from build123d import *
from OCP.BRepFilletAPI import BRepFilletAPI_MakeChamfer

# Parameters (mm, degrees)
SKETCH_1_W      = 20.2
SKETCH_1_H      = 50
SKETCH_1_R      = 1.325
SKETCH_1_R_2    = 1.595
SKETCH_1_W_2    = 6
SKETCH_1_H_2    = 10.9
EXTRUDE_1_DEPTH = 2
FILLET_1_R      = 2
CHAMFER_1_SIZE  = 0.6
CHAMFER_2_SIZE  = 0.5
CHAMFER_2_SIZE2 = 0.595876796


with BuildPart() as part:
    # 草图1 → 凸台-拉伸1 (new body)
    with BuildSketch(Plane.XY):
        with Locations((-6.4, 0)):
            Rectangle(SKETCH_1_W, SKETCH_1_H)
        with Locations((-14.25, -22.65)):
            Circle(SKETCH_1_R, mode=Mode.SUBTRACT)
        with Locations((-14.25, 22.65)):
            Circle(SKETCH_1_R, mode=Mode.SUBTRACT)
        with Locations((1.45, 22.65)):
            Circle(SKETCH_1_R, mode=Mode.SUBTRACT)
        with Locations((1.45, -22.65)):
            Circle(SKETCH_1_R, mode=Mode.SUBTRACT)
        with Locations((-10.36, -6.365)):
            Circle(SKETCH_1_R_2, mode=Mode.SUBTRACT)
        with Locations((-10.36, -11.8216)):
            Circle(SKETCH_1_R_2, mode=Mode.SUBTRACT)
        with Locations((-4.095, 6)):
            Rectangle(SKETCH_1_W_2, SKETCH_1_H_2, mode=Mode.SUBTRACT)
    extrude(amount=EXTRUDE_1_DEPTH)

    # 圆角1
    fillet_1_edges = [part.edges().sort_by_distance(p)[0] for p in [
        (-16.5, 25, 1),
        (3.7, 25, 1),
        (3.7, -25, 1),
        (-16.5, -25, 1),
    ]]
    fillet(fillet_1_edges, radius=FILLET_1_R)

    # 倒角1
    chamfer_1_edges = [part.edges().sort_by_distance(p)[0] for p in [
        (-15.575, -22.65, 2),
        (-15.575, 22.65, 2),
        (0.125, 22.65, 2),
        (0.125, -22.65, 2),
    ]]
    chamfer(chamfer_1_edges, length=CHAMFER_1_SIZE)

    # 倒角2: one chamfer whose edges measure the first distance from different faces: ONE call of the kernel's chamfer builder (chamfer() names one face for all edges)
    chamfer_2_edges_1 = [part.edges().sort_by_distance(p)[0] for p in [
        (-7.095, 6, 0),
        (-7.095, 11.45, 1),
        (-7.095, 0.55, 1),
        (-7.095, 6, 2),
    ]]
    chamfer_2_side_1 = [part.faces().sort_by_distance(p)[0] for p in [
        (-7.095, 6, 1),
    ]]
    chamfer_2_edges_2 = [part.edges().sort_by_distance(p)[0] for p in [
        (-4.095, 0.55, 0),
    ]]
    chamfer_2_side_2 = [part.faces().sort_by_distance(p)[0] for p in [
        (-4.095, 0.55, 1),
    ]]
    chamfer_2_edges_3 = [part.edges().sort_by_distance(p)[0] for p in [
        (-1.095, 6, 0),
        (-1.095, 0.55, 1),
    ]]
    chamfer_2_side_3 = [part.faces().sort_by_distance(p)[0] for p in [
        (-1.095, 6, 1),
    ]]
    chamfer_2_edges_4 = [part.edges().sort_by_distance(p)[0] for p in [
        (-4.095, 11.45, 0),
        (-1.095, 11.45, 1),
    ]]
    chamfer_2_side_4 = [part.faces().sort_by_distance(p)[0] for p in [
        (-4.095, 11.45, 1),
    ]]
    chamfer_2_edges_5 = [part.edges().sort_by_distance(p)[0] for p in [
        (-4.095, 0.55, 2),
        (-1.095, 6, 2),
        (-4.095, 11.45, 2),
    ]]
    chamfer_2_side_5 = [part.faces().sort_by_distance(p)[0] for p in [
        (-6.499529382, -0.281178063, 2),
    ]]
    chamfer_2 = BRepFilletAPI_MakeChamfer(part.part.solid().wrapped)
    for e in chamfer_2_edges_1:
        chamfer_2.Add(CHAMFER_2_SIZE, CHAMFER_2_SIZE2, e.wrapped, chamfer_2_side_1[0].wrapped)  # the first distance lies on this face
    for e in chamfer_2_edges_2:
        chamfer_2.Add(CHAMFER_2_SIZE, CHAMFER_2_SIZE2, e.wrapped, chamfer_2_side_2[0].wrapped)  # the first distance lies on this face
    for e in chamfer_2_edges_3:
        chamfer_2.Add(CHAMFER_2_SIZE, CHAMFER_2_SIZE2, e.wrapped, chamfer_2_side_3[0].wrapped)  # the first distance lies on this face
    for e in chamfer_2_edges_4:
        chamfer_2.Add(CHAMFER_2_SIZE, CHAMFER_2_SIZE2, e.wrapped, chamfer_2_side_4[0].wrapped)  # the first distance lies on this face
    for e in chamfer_2_edges_5:
        chamfer_2.Add(CHAMFER_2_SIZE, CHAMFER_2_SIZE2, e.wrapped, chamfer_2_side_5[0].wrapped)  # the first distance lies on this face
    add(Compound.cast(chamfer_2.Shape()), mode=Mode.REPLACE)


solid = part.part
Here's how the part is built. I have some questions about the finished solid (model axes, mm). A direction names the side the tool comes from. Round coordinates to 2 decimals unless told otherwise and drop trailing zeros. Order: outer loops, then holes, each group sorted by start corner. A loop starts at its lowest first (then second) coordinate and runs counter-clockwise, first axis right, second up. Notation, with made-up numbers: (89.25, -40) -> (126.25, -40) arc R11 cw to (126.25, -26) -> close; hole circle Ø6 at (33.25, 49.25). An arc over 180 degrees is marked (long way). Use CSV: the item, a comma, the result in double quotes.
1. I'm going to push a flat-ended pin straight in: P1, Ø3.5, axis at x = 1.45, y = -22.65, coming from the +Z side (3 decimals). Where does the tip first touch, or does it pass through?
Recorded:
P1,"stops at z = 1.825"
2. I need wall thicknesses on line 1 along Y through (x, z) = (-10.36, 1.3); line 2 along Y through (x, z) = (-14.25, 1.1) (3 decimals); line 3 along Y through (x, z) = (-4.75, 0.65). Which ranges of each line are inside material? Lowest first, please.
Recorded:
line 1,"y = -25 to -13.42, -10.23 to -7.96, -4.77 to 25"
line 2,"y = -25 to -23.975, -21.325 to 21.325, 23.975 to 25"
line 3,"y = -25 to 0.55, 11.45 to 25"
3. I want a section at A-A on x = -10.36. List the corners of the cut face in (y, z) for me, and give its area (3 significant figures).
Recorded:
outline,"(-25, 0) -> (-13.42, 0) -> (-13.42, 2) -> (-25, 2) -> close; (-10.23, 0) -> (-7.96, 0) -> (-7.96, 2) -> (-10.23, 2) -> close; (-4.77, 0) -> (25, 0) -> (25, 2) -> (-4.77, 2) -> close"
area,"87.2 mm2"
4. Thinking about a two-plate mould opening in Y: for faces 1 (the face through (1.278, -21.336, 0.69)), 2 (the face through (-9, 0, 0)), 3 (the face through (-15.93, -24.4, 1.01)), 4 (the face through (-15.93, 24.4, 1.01)), which applies, pulls with the +Y half, pulls with the -Y half, needs draft (parallel to the pull), parting line crosses it, or undercut?
Recorded:
face 1,"undercut"
face 2,"needs draft"
face 3,"pulls with the -Y half"
face 4,"pulls with the +Y half"
5. I want a section at B-B on y = 3. List the corners of the cut face in (x, z) for me (3 decimals), and give its area (3 significant figures).
Recorded:
outline,"(-16.5, 0) -> (-7.691, 0) -> (-7.095, 0.5) -> (-7.095, 1.5) -> (-7.691, 2) -> (-16.5, 2) -> close; (-1.095, 0.5) -> (-0.499, 0) -> (3.7, 0) -> (3.7, 2) -> (-0.595, 2) -> (-1.095, 1.404) -> close"
area,"27.8 mm2"
6. I want a section at C-C on z = 0.95. List the corners of the cut face in (x, y) for me (3 decimals), and give its area (3 significant figures).
Recorded:
outline,"(-16.5, -23) arc R2 ccw to (-14.5, -25) -> (1.7, -25) arc R2 ccw to (3.7, -23) -> (3.7, 23) arc R2 ccw to (1.7, 25) -> (-14.5, 25) arc R2 ccw to (-16.5, 23) -> close; hole circle Ø2.65 at (-14.25, -22.65); hole circle Ø2.65 at (-14.25, 22.65); hole circle Ø3.19 at (-10.36, -11.822); hole circle Ø3.19 at (-10.36, -6.365); hole (-7.095, 1.05) -> (-6.499, 0.55) -> (-1.691, 0.55) -> (-1.095, 1.05) -> (-1.095, 10.854) -> (-1.595, 11.45) -> (-6.499, 11.45) -> (-7.095, 10.95) -> close; hole circle Ø2.65 at (1.45, -22.65); hole circle Ø2.65 at (1.45, 22.65)"
area,"904 mm2"
7. Which directions (+Z, -Z, +X, -X, +Y, -Y) give clear straight access to the entire face, cutting with the end or side of a thin tool? Please do faces 5 (the face through (-4, 0.55, 1)), 6 (the face through (3.1, -24.43, 1.01)).
Recorded:
face 5,"+Z, -Z"
face 6,"+Z, -Z, +X, -Y"
